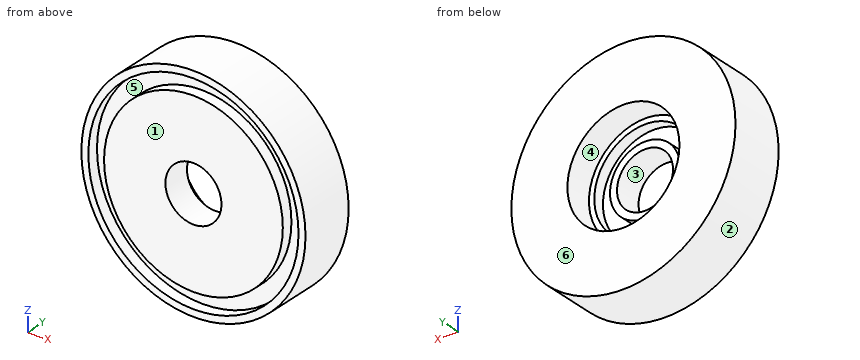
```python
from build123d import *


with BuildPart() as part:
    # Sketch1 → Revolve1 (revolve)
    with BuildSketch(Plane.XY):
        Polygon((-6.35, 0), (-6.35, 6.35), (-7.9375, 6.35), (-7.9375, 3.81), (-11.4935, 3.81), (-11.4935, 6.35), (-12.7, 6.35), (-12.7, 12.7), (-25.4, 12.7), (-25.4, 0), (-23.8125, 0), (-23.8125, 2.54), (-20.2565, 2.54), (-20.2565, 0), align=None)
    revolve(axis=Axis((0, 0, 0), (0, 1, 0)))


solid = part.part
```
Check sheet for the modelled part. Datum: model origin and axes. Units: mm. Face numbers are marked on the shaded views. A direction names the side the tool comes from. Give positions to 0.01 mm unless a question says otherwise; leave off trailing zeros. Order: outer loops, then holes, each group sorted by start corner. A loop starts at its lowest first (then second) coordinate and runs counter-clockwise, first axis right, second up. Notation, with made-up numbers: M -25.5,2 L 4.5,2 A26 cw 4.5,27 Z; hole C 83,73.25 d3. An arc over 180 degrees is marked long. Answer in a Markdown table with one row per item.
1) Gauge pin test, flat ends, axial feed: P1, Ø1, axis at y = 1.5, z = 19.5, coming from the -X side; P2, Ø3, axis at y = 10.5, z = -12.5, coming from the +X side; P3, Ø12.5, axis at x = -1, z = -1.5, coming from the +Y side. Record the tip position at first contact, or that the pin passes through.
Filled sheet:
| item | result |
|---|---|
| P1 | stops at x = -16.86 |
| P2 | stops at x = 22.89 |
| P3 | stops at y = 6.35 |
2) Access from +Z, -Z, +X, -X, +Y, -Y to the whole of each face (thin tool, end or side, straight path). Record for the marked faces 4, 5 and 6.
Filled sheet:
| item | result |
|---|---|
| face 4 | +Y |
| face 5 | -Y |
| face 6 | +Z, -Z, +X, -X, +Y |
3) Cross-section at C-C, the plane y = 7.5. Enter the section's corners in (x, z), plus the area to 3 significant figures.
Filled sheet:
| item | result |
|---|---|
| outline | C 0,0 d50.8; hole C 0,0 d25.4 |
| area | 1,520 mm2 |
4) Cross-section at B-B, the plane x = 0. Enter the section's corners in (y, z).
Filled sheet:
| item | result |
|---|---|
| outline | M 0,-25.4 L 12.7,-25.4 L 12.7,-12.7 L 6.35,-12.7 L 6.35,-11.49 L 3.81,-11.49 L 3.81,-7.94 L 6.35,-7.94 L 6.35,-6.35 L 0,-6.35 L 0,-20.26 L 2.54,-20.26 L 2.54,-23.81 L 0,-23.81 Z; M 0,6.35 L 6.35,6.35 L 6.35,7.94 L 3.81,7.94 L 3.81,11.49 L 6.35,11.49 L 6.35,12.7 L 12.7,12.7 L 12.7,25.4 L 0,25.4 L 0,23.81 L 2.54,23.81 L 2.54,20.26 L 0,20.26 Z |
5) Release check for a two-part mould opening along X. For the marked faces 1, 2 and 3 record: +X half, -X half, draft (parallel to the pull), parting line (faces both ways), or undercut.
Filled sheet:
| item | result |
|---|---|
| face 1 | draft |
| face 2 | parting line |
| face 3 | undercut |
6) Cross-section at D-D, the plane z = 22. Enter the section's corners in (x, y), plus the area to 3 significant figures.
Filled sheet:
| item | result |
|---|---|
| outline | M -12.69,0 L -9.11,0 L -9.11,2.54 L 9.11,2.54 L 9.11,0 L 12.69,0 L 12.69,12.7 L -12.69,12.7 Z |
| area | 276 mm2 |
7) Thickness scan on L1, parallel to Z at x = 0, y = 1.95; L2, parallel to X at y = 5.25, z = -2.5; L3, parallel to X at y = 1.5, z = 11.5. Record the ranges inside material, lowest first. Write a range as [from, to].
Filled sheet:
| item | result |
|---|---|
| L1 | z = [-25.4, -23.81], [-20.26, -6.35], [6.35, 20.26], [23.81, 25.4] |
| L2 | x = [-25.28, -11.22], [-7.53, -5.84], [5.84, 7.53], [11.22, 25.28] |
| L3 | x = [-22.65, -20.85], [-16.68, 16.68], [20.85, 22.65] |
8) Cross-section at A-A, the plane z = 0. Enter the section's corners in (x, y).
Filled sheet:
| item | result |
|---|---|
| outline | M -25.4,0 L -23.81,0 L -23.81,2.54 L -20.26,2.54 L -20.26,0 L -6.35,0 L -6.35,6.35 L -7.94,6.35 L -7.94,3.81 L -11.49,3.81 L -11.49,6.35 L -12.7,6.35 L -12.7,12.7 L -25.4,12.7 Z; M 6.35,0 L 20.26,0 L 20.26,2.54 L 23.81,2.54 L 23.81,0 L 25.4,0 L 25.4,12.7 L 12.7,12.7 L 12.7,6.35 L 11.49,6.35 L 11.49,3.81 L 7.94,3.81 L 7.94,6.35 L 6.35,6.35 Z |
